```python
from build123d import *

# Parameters (mm, degrees)
SKETCH1_W           = 43
SKETCH1_H           = 43
BOSS_EXTRUDE1_DEPTH = 38
SKETCH3_R           = 3
SKETCH3_R_2         = 7.25
CUT_EXTRUDE4_DEPTH  = 38
SKETCH6_W           = 39
SKETCH6_H           = 39
CUT_EXTRUDE5_DEPTH  = 22
CUT_EXTRUDE8_START  = -12
SKETCH7_W           = 43
SKETCH7_H           = 43
SKETCH7_R           = 3
SKETCH7_W_2         = 18.4
SKETCH7_H_2         = 18.4
CUT_EXTRUDE8_DEPTH  = 12
FILLET2_R           = 5
FILLET3_R           = 3


with BuildPart() as part:
    # Sketch1 → Boss-Extrude1 (new body)
    with BuildSketch(Plane(origin=(0, 0, 0), x_dir=(0, 1, 0), z_dir=(0, 0, 1))):
        with Locations((-19.5, 19.5)):
            Rectangle(SKETCH1_W, SKETCH1_H)
    extrude(amount=BOSS_EXTRUDE1_DEPTH)

    # Sketch3 → Cut-Extrude4 (cut)
    with BuildSketch(Plane.XY.offset(38)):
        with Locations((-20, -3.506761261)):
            Circle(SKETCH3_R)
        with Locations((-20, -19)):
            Circle(SKETCH3_R_2)
        with BuildLine():
            Line((-6, -13), (-6, -25))
            ThreePointArc((-6, -25), (-3, -28), (0, -25))
            Line((0, -25), (0, -13))
            ThreePointArc((0, -13), (-3, -10), (-6, -13))
        make_face()
        with BuildLine():
            Line((-33, -13), (-33, -25))
            ThreePointArc((-33, -25), (-36, -28), (-39, -25))
            Line((-39, -25), (-39, -13))
            ThreePointArc((-39, -13), (-36, -10), (-33, -13))
        make_face()
    extrude(amount=-CUT_EXTRUDE4_DEPTH, mode=Mode.SUBTRACT)

    # Sketch6 → Cut-Extrude5 (cut)
    with BuildSketch(Plane.XY.offset(38)):
        with Locations((-19.5, -19.5)):
            Rectangle(SKETCH6_W, SKETCH6_H)
    extrude(amount=-CUT_EXTRUDE5_DEPTH, mode=Mode.SUBTRACT)

    # Sketch7 → Cut-Extrude8 (cut)
    with BuildSketch(Plane(origin=(0, 0, 0), x_dir=(1, 0, 0), z_dir=(0, 0, -1)).offset(CUT_EXTRUDE8_START)):
        with Locations((-19.5, 19.5)):
            Rectangle(SKETCH7_W, SKETCH7_H)
        with Locations((-20, 3.506761261)):
            Circle(SKETCH7_R, mode=Mode.SUBTRACT)
        with Locations((-20.012556467, 19.015852406)):
            Rectangle(SKETCH7_W_2, SKETCH7_H_2, mode=Mode.SUBTRACT)
        with BuildLine():
            Line((-33, 25), (-33, 13))
            ThreePointArc((-33, 13), (-36, 10), (-39, 13))
            Line((-39, 13), (-39, 25))
            ThreePointArc((-39, 25), (-36, 28), (-33, 25))
        make_face(mode=Mode.SUBTRACT)
        with BuildLine():
            ThreePointArc((0, 13), (-3, 10), (-6, 13))
            Line((-6, 13), (-6, 25))
            ThreePointArc((-6, 25), (-3, 28), (0, 25))
            Line((0, 25), (0, 13))
        make_face(mode=Mode.SUBTRACT)
    extrude(amount=CUT_EXTRUDE8_DEPTH, mode=Mode.SUBTRACT)

    # Fillet2
    fillet2_edges = [part.edges().sort_by_distance(p)[0] for p in [
        (-10.812556467, -9.815852406, 6),
        (-10.812556467, -28.215852406, 6),
        (-29.212556467, -28.215852406, 6),
        (-29.212556467, -9.815852406, 6),
    ]]
    fillet(fillet2_edges, radius=FILLET2_R)

    # Fillet3
    fillet3_edges = [part.edges().sort_by_distance(p)[0] for p in [
        (-41, -41, 25),
        (2, -41, 25),
        (2, 2, 25),
        (-41, 2, 25),
    ]]
    fillet(fillet3_edges, radius=FILLET3_R)


solid = part.part
```
The model under review builds one solid part; all positions refer to its coordinate system, in mm. A direction names the side the tool comes from. Round coordinates to 2 decimals unless told otherwise and drop trailing zeros. Loops run counter-clockwise (first coordinate to the right, second up) from the corner with the lowest first, then second, coordinate; pieces in that order, holes last. Notation, with made-up numbers: (55, -13) - (61, -13) arc R30 cw to (61, 14) - close; hole circle Ø10 at (82.25, 67.25). An arc over 180 degrees is marked (long way). Use a Markdown table: item, result. Add a question column.
Q1. For probe 1 along Y at (x, z) = (-20, 13); probe 2 along Y at (x, z) = (-20, 7.5); probe 3 along X at (y, z) = (-33, 21), list the stretches that pass through material, from the lowest coordinate up.
Q2. Insertion check: pin 1 Ø6 at (x, z) = (-27.5, 5.5) entering from -Y; pin 2 Ø1 at (x, y) = (-10.5, -24) entering from +Z; pin 3 Ø4 at (x, z) = (-19, 4.5) entering from +Y. Each pin has a flat end and moves straight along its axis. Give the tip position at first contact, or say it passes through.
Q3. Add section D-D (x = -20). State the section outline as (y, z) points, plus the area to 3 significant figures.
Q4. Machinability: for faces 1 (the face through (-12.238, -26.712, 5.916)), 2 (the face through (-27.8, -26.7, 5.9)), 3 (the face through (0, -20, 25)), which of the approach directions +Z, -Z, +X, -X, +Y, -Y give a long, thin tool a straight path to every point of the face, cutting with its end or side? Answer none if there is none.
Q5. The part is to be moulded in two halves that separate along X. For faces 4 (the face through (-20, -9.816, 6)), 5 (the face through (1.1, -40.14, 25.18)), 6 (the face through (-23, -3.4, 14)), say which applies: pulls with the +X half, pulls with the -X half, needs draft (parallel to the pull), parting line crosses it, or undercut.
Q6. Add section A-A (x = -36). State the section outline as (y, z) points.
Q7. Add section B-B (y = -19). State the section outline as (x, z) points, plus the area to 3 significant figures.
Q8. Add section C-C (z = 31.5). State the section outline as (x, y) points.
Worked answers:
| question | item | result |
|---|---|---|
| 1 | probe 1 | -41 to -26.25, -11.75 to -6.51, -0.51 to 2 |
| 1 | probe 2 | -28.22 to -26.25, -11.75 to -9.82 |
| 1 | probe 3 | -41 to -39, 0 to 2 |
| 2 | pin 1 | y = -28.21 |
| 2 | pin 2 | z = 16 |
| 2 | pin 3 | y = -9.82 |
| 3 | outline | (-41, 12) - (-28.22, 12) - (-28.22, 0) - (-26.25, 0) - (-26.25, 16) - (-39, 16) - (-39, 38) - (-41, 38) - close; (-11.75, 0) - (-9.82, 0) - (-9.82, 12) - (-6.51, 12) - (-6.51, 16) - (-11.75, 16) - close; (-0.51, 12) - (2, 12) - (2, 38) - (0, 38) - (0, 16) - (-0.51, 16) - close |
| 3 | area | 225 mm² |
| 4 | face 1 | -Z, +X, -Y |
| 4 | face 2 | -Z, -X, -Y |
| 4 | face 3 | +Z |
| 5 | face 4 | needs draft |
| 5 | face 5 | pulls with the +X half |
| 5 | face 6 | undercut |
| 6 | outline | (-41, 12) - (-28, 12) - (-28, 16) - (-39, 16) - (-39, 38) - (-41, 38) - close; (-10, 12) - (2, 12) - (2, 38) - (0, 38) - (0, 16) - (-10, 16) - close |
| 7 | outline | (-41, 12) - (-39, 12) - (-39, 38) - (-41, 38) - close; (-33, 12) - (-29.21, 12) - (-29.21, 0) - (-27.25, 0) - (-27.25, 16) - (-33, 16) - close; (-12.75, 0) - (-10.81, 0) - (-10.81, 12) - (-6, 12) - (-6, 16) - (-12.75, 16) - close; (0, 12) - (2, 12) - (2, 38) - (0, 38) - close |
| 7 | area | 201 mm² |
| 8 | outline | (-41, -38) arc R3 ccw to (-38, -41) - (-1, -41) arc R3 ccw to (2, -38) - (2, -1) arc R3 ccw to (-1, 2) - (-38, 2) arc R3 ccw to (-41, -1) - close; hole (-39, -39) - (0, -39) - (0, 0) - (-39, 0) - close |
